Source: CAD feature listing. Evaluate the final solid. Frame: model axes, mm. Face numbers are marked on the shaded views. Coordinates: 2 decimals unless noted, no trailing zeros. Loops run counter-clockwise (first coordinate to the right, second up) from the corner with the lowest first, then second, coordinate; pieces in that order, holes last.
Item 1: Section query C-C, the plane x = 0. State how many separate pieces and enclosed holes the cut face has, then the cut area to 3 significant figures.
Item 2: Pull-direction query (X, two-part tool) for the marked faces 1 and 2; classes: +X half, -X half, draft (parallel to the pull), parting line (faces both ways), or undercut.
Item 3: Line query: probe 1 along X at (y, z) = (-13.5, 2.9); probe 2 along Y at (x, z) = (0, 3.4); probe 3 along Y at (x, z) = (-23, 3.55). Output: solid intervals per line, ascending.
Item 4: Section query B-B, the plane y = 29.5. Return the cut outline in (x, z), then the cut area to 3 significant figures.
Item 5: Section query A-A, the plane x = -11.5. Return the cut outline in (y, z).
Item 6: Section query D-D, the plane y = -22. Return the cut outline in (x, z).
Item 7: Pin query (flat end, axial travel): pin 1 Ø8 at (x, y) = (-11.5, -28.5) entering from -Z. Return the tip coordinate at first contact, or that it passes through.
```python
from build123d import *

# Parameters (mm, degrees)
F0_W      = 60
F0_H      = 93
F0_W_2    = 54
F0_H_2    = 87
F1_DEPTH  = 3
F2_W      = 60
F2_H      = 93
F2_W_2    = 5
F2_H_2    = 30
F3_DEPTH  = 2
F5_DEPTH  = 5
F7_DEPTH  = 5
F8_W      = 54
F8_H      = 1.5
F9_DEPTH  = 5
F11_DEPTH = 54
F12_R     = 3.152698
F12_R_2   = 3
F13_DEPTH = 25


with BuildPart() as f1:
    # F0 (on Top) → F1 (new body)
    with BuildSketch(Plane.XY):
        Rectangle(F0_W, F0_H)
        Rectangle(F0_W_2, F0_H_2, mode=Mode.SUBTRACT)
    extrude(amount=F1_DEPTH)

    # F2 (on face) → F3 (join)
    with BuildSketch(Plane.XY.offset(3)):
        Rectangle(F2_W, F2_H)
        with Locations((-20, 0)):
            Rectangle(F2_W_2, F2_H_2, mode=Mode.SUBTRACT)
        with BuildLine():
            Line((-5, 25), (5, 25))
            ThreePointArc((5, 25), (8.535534, 23.535534), (10, 20))
            Line((10, 20), (10, -20))
            ThreePointArc((10, -20), (8.535534, -23.535534), (5, -25))
            Line((5, -25), (-5, -25))
            ThreePointArc((-5, -25), (-8.535534, -23.535534), (-10, -20))
            Line((-10, -20), (-10, 20))
            ThreePointArc((-10, 20), (-8.535534, 23.535534), (-5, 25))
        make_face(mode=Mode.SUBTRACT)
        with Locations((20, 0)):
            Rectangle(F2_W_2, F2_H_2, mode=Mode.SUBTRACT)
    extrude(amount=F3_DEPTH)

    # F4 (on face) → F5 (join)
    with BuildSketch(Plane(origin=(-17.5, 0, 0), x_dir=(0, -1, 0), z_dir=(-1, 0, 0))):
        Polygon((15, 3), (15, 5), (-15, 2.111329), (-15, 0.111329), align=None)
    extrude(amount=F5_DEPTH)

    # F6 (on face) → F7 (join)
    with BuildSketch(Plane.YZ.offset(17.5)):
        Polygon((15, 2.111329), (-15, 5), (-15, 3), (15, 0.111329), align=None)
    extrude(amount=F7_DEPTH)

    # F8 (on face) → F9 (cut)
    with BuildSketch(Plane.XZ.offset(46.5)):
        with Locations((0, 2)):
            Rectangle(F8_W, F8_H)
    extrude(amount=-F9_DEPTH, mode=Mode.SUBTRACT)

    # F10 (on face) → F11 (join, through all)
    with BuildSketch(Plane(origin=(27, 0, 0), x_dir=(0, -1, 0), z_dir=(-1, 0, 0))):
        Polygon((43.5, 0), (43.5, 1.25), (42.25, 0), align=None)
    extrude(amount=F11_DEPTH)

    # F12 (on face) → F13 (cut)
    with BuildSketch(Plane.XY.offset(5)):
        with Locations((-23, 39.5)):
            Circle(F12_R)
        with Locations((-23, 29.5)):
            Circle(F12_R)
        with Locations((-11.5, 39.5)):
            Circle(F12_R)
        with Locations((-11.5, 29.5)):
            Circle(F12_R)
        with Locations((0, 39.5)):
            Circle(F12_R)
        with Locations((0, 29.5)):
            Circle(F12_R)
        with Locations((11.5, 39.5)):
            Circle(F12_R)
        with Locations((11.5, 29.5)):
            Circle(F12_R)
        with Locations((23, 39.5)):
            Circle(F12_R)
        with Locations((23, 29.5)):
            Circle(F12_R)
        with Locations((-23, -38.5)):
            Circle(F12_R_2)
        with Locations((-23, -28.5)):
            Circle(F12_R_2)
        with Locations((-11.5, -38.5)):
            Circle(F12_R_2)
        with Locations((-11.5, -28.5)):
            Circle(F12_R_2)
        with Locations((0, -38.5)):
            Circle(F12_R_2)
        with Locations((0, -28.5)):
            Circle(F12_R_2)
        with Locations((11.5, -38.5)):
            Circle(F12_R_2)
        with Locations((11.5, -28.5)):
            Circle(F12_R_2)
        with Locations((23, -38.5)):
            Circle(F12_R_2)
        with Locations((23, -28.5)):
            Circle(F12_R_2)
    extrude(amount=-F13_DEPTH, mode=Mode.SUBTRACT)


solid = f1.part
```
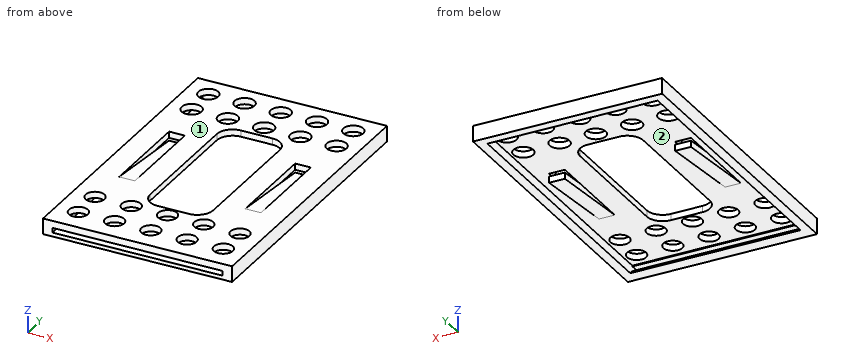
Verdict:
1. separate pieces: 7
1. enclosed holes: 0
1. area: 51.1 mm2
2. face 1: draft
2. face 2: undercut
3. probe 1: x = -30 to -27, -22.5 to -17.5, 17.5 to 22.5, 27 to 30
3. probe 2: y = -46.5 to -41.5, -35.5 to -31.5, -25.5 to -25, 25 to 26.35, 32.65 to 36.35, 42.65 to 46.5
3. probe 3: y = -46.5 to -41.5, -35.5 to -31.5, -25.5 to 26.35, 32.65 to 36.35, 42.65 to 46.5
4. outline: (-30, 0) - (-27, 0) - (-27, 3) - (-26.15, 3) - (-26.15, 5) - (-30, 5) - close; (-19.85, 3) - (-14.65, 3) - (-14.65, 5) - (-19.85, 5) - close; (-8.35, 3) - (-3.15, 3) - (-3.15, 5) - (-8.35, 5) - close; (3.15, 3) - (8.35, 3) - (8.35, 5) - (3.15, 5) - close; (14.65, 3) - (19.85, 3) - (19.85, 5) - (14.65, 5) - close; (26.15, 3) - (27, 3) - (27, 0) - (30, 0) - (30, 5) - (26.15, 5) - close
4. area: 74.9 mm2
5. outline: (-46.5, 0) - (-42.25, 0) - (-43.5, 1.25) - (-46.5, 1.25) - close; (-46.5, 2.75) - (-43.5, 2.75) - (-43.5, 3) - (-41.5, 3) - (-41.5, 5) - (-46.5, 5) - close; (-35.5, 3) - (-31.5, 3) - (-31.5, 5) - (-35.5, 5) - close; (-25.5, 3) - (26.35, 3) - (26.35, 5) - (-25.5, 5) - close; (32.65, 3) - (36.35, 3) - (36.35, 5) - (32.65, 5) - close; (42.65, 3) - (43.5, 3) - (43.5, 0) - (46.5, 0) - (46.5, 5) - (42.65, 5) - close
6. outline: (-30, 0) - (-27, 0) - (-27, 3) - (-9.58, 3) - (-9.58, 5) - (-30, 5) - close; (9.58, 3) - (27, 3) - (27, 0) - (30, 0) - (30, 5) - (9.58, 5) - close
7. pin 1: stops at z = 3
